Design review of the part built by this model. Coordinates are the model's own, in mm. Give positions to 0.01 mm unless a question says otherwise; leave off trailing zeros. Write each loop counter-clockwise with the first axis right and the second up, starting at its lowest first coordinate (ties: lowest second). Pieces come first, ordered by that corner, then holes. Notation, with made-up numbers: (37, 51) - (75, 51) arc R25 ccw to (75, 83) - close; hole circle Ø7 at (70.25, -7.5). An arc over 180 degrees is marked (long way). Use a Markdown table: item, result. Add a question column.
```python
from build123d import *

# Parameters (mm, degrees)
CROQUIS2_R                = 4.7625
SALIENTE_EXTRUIR1_DEPTH   = 45.24375
CHAFL_N1_SIZE             = 0.396875
CROQUIS4_R                = 2.4892
CLEARANCE_HOLE_DEPTH      = 46.24375
CLEARANCE_HOLE_DEPTH_BACK = 46.24375


with BuildPart() as part:
    # Croquis2 → Saliente-Extruir1 (new body, symmetric)
    with BuildSketch(Plane(origin=(0, 0, 0), x_dir=(1, 0, 0), z_dir=(0, 1, 0))):
        Circle(CROQUIS2_R)
    extrude(amount=SALIENTE_EXTRUIR1_DEPTH, both=True)

    # Chafl_n1
    chafl_n1_edges = [part.edges().sort_by_distance(p)[0] for p in [
        (-4.7625, -45.24375, 0),
        (-4.7625, 45.24375, 0),
    ]]
    chamfer(chafl_n1_edges, length=CHAFL_N1_SIZE)

    # Croquis4 → Clearance Hole (cut, two sides)
    with BuildSketch(Plane(origin=(0, 0, 0), x_dir=(1, 0, 0), z_dir=(0, 1, 0))) as clearance_hole_sk:
        Circle(CROQUIS4_R)
    extrude(amount=CLEARANCE_HOLE_DEPTH, mode=Mode.SUBTRACT)
    extrude(clearance_hole_sk.sketch, amount=-CLEARANCE_HOLE_DEPTH_BACK, mode=Mode.SUBTRACT)


solid = part.part
```
(1) Add section A-A (x = 0). State the section outline as (y, z) points.
(2) Mouldability with a two-part tool opening along X and no side actions: class faces 1 (the face through (-3.78, 0.63, 2.9)), 2 (the face through (2.374, 0.633, -0.748)), 3 (the face through (2, 45.244, 2)) as +X half, -X half, draft (parallel to the pull), parting line (faces both ways), or undercut.
(3) For line 1 along X through (y, z) = (-19, 0); line 2 along Z through (x, y) = (-2, 13.5), list the stretches that pass through material, from the lowest coordinate up.
(4) Insertion check: pin 1 (4 mm diameter, centred on x = -2.5, y = 31, fed in from -Z). The pin has a flat end and moves straight along its axis. Give the tip position at first contact, or say it passes through.
(5) Add section B-B (y = 33.5). State the section outline as (x, z) points (1 decimal).
Answers follow:
| question | item | result |
|---|---|---|
| 1 | outline | (-45.24, -4.37) - (-44.85, -4.76) - (44.85, -4.76) - (45.24, -4.37) - (45.24, -2.49) - (-45.24, -2.49) - close; (-45.24, 2.49) - (45.24, 2.49) - (45.24, 4.37) - (44.85, 4.76) - (-44.85, 4.76) - (-45.24, 4.37) - close |
| 2 | face 1 | parting line |
| 2 | face 2 | undercut |
| 2 | face 3 | draft |
| 3 | line 1 | -4.76 to -2.49, 2.49 to 4.76 |
| 3 | line 2 | -4.32 to -1.48, 1.48 to 4.32 |
| 4 | pin 1 | z = -4.74 |
| 5 | outline | circle Ø9.5 at (0, 0); hole circle Ø5 at (0, 0) |
